Design review of the part built by this model. Coordinates are the model's own, in mm. Face numbers are marked on the shaded views. A direction names the side the tool comes from. Coordinates: 2 decimals unless noted, no trailing zeros. Loops run counter-clockwise (first coordinate to the right, second up) from the corner with the lowest first, then second, coordinate; pieces in that order, holes last. Notation, with made-up numbers: M -21.5,-23.75 L 34.5,-23.75 A21 cw 34.5,15.25 Z; hole C 23.5,5 d6. An arc over 180 degrees is marked long. One line per item, written item: value.
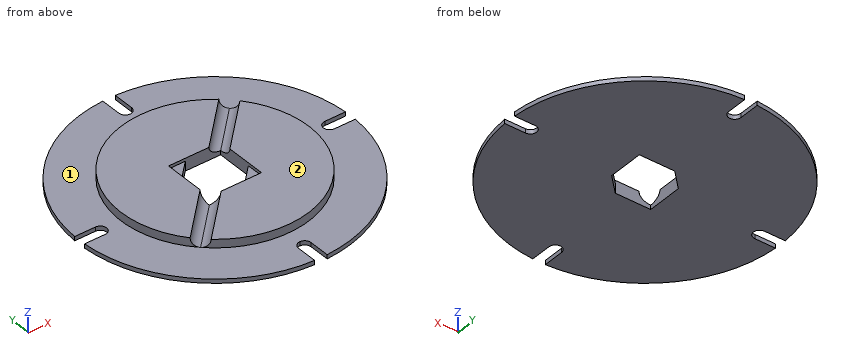
```python
from build123d import *

# Parameters (mm, degrees)
F2_DEPTH      = 2
F3_DEPTH      = 6
F4_DEPTH      = 6
F5_DEPTH      = 4.6
F9_DEPTH      = 45
F9_DEPTH_BACK = 45


with BuildPart() as f2:
    # F0 (on Top) → F2 (new body)
    with BuildSketch(Plane.XY):
        with BuildLine():
            Line((55, 3), (64.930732323, 3))
            ThreePointArc((64.930732323, 3), (45.9619407771, 45.9619407771), (3, 64.930732323))
            Line((3, 64.930732323), (3, 55))
            ThreePointArc((3, 55), (0, 52), (-3, 55))
            Line((-3, 55), (-3, 64.930732323))
            ThreePointArc((-3, 64.930732323), (-45.9619407771, 45.9619407771), (-64.930732323, 3))
            Line((-64.930732323, 3), (-55, 3))
            ThreePointArc((-55, 3), (-52, 0), (-55, -3))
            Line((-55, -3), (-64.930732323, -3))
            ThreePointArc((-64.930732323, -3), (-45.9619407771, -45.9619407771), (-3, -64.930732323))
            Line((-3, -64.930732323), (-3, -55))
            ThreePointArc((-3, -55), (-2.1213203436, -52.8786796564), (0, -52))
            ThreePointArc((0, -52), (2.1213203436, -52.8786796564), (3, -55))
            Line((3, -55), (3, -64.930732323))
            ThreePointArc((3, -64.930732323), (45.9619407771, -45.9619407771), (64.930732323, -3))
            Line((64.930732323, -3), (55, -3))
            ThreePointArc((55, -3), (52, 0), (55, 3))
        make_face()
        with BuildLine():
            ThreePointArc((45, 0), (31.8198051534, -31.8198051534), (0, -45))
            ThreePointArc((0, -45), (-31.8198051534, 31.8198051534), (45, 0))
        make_face(mode=Mode.SUBTRACT)
    extrude(amount=F2_DEPTH)

    # F0 (on Top) → F3 (join)
    with BuildSketch(Plane.XY):
        with BuildLine():
            ThreePointArc((45, 0), (-31.8198051534, 31.8198051534), (0, -45))
            ThreePointArc((0, -45), (31.8198051534, -31.8198051534), (45, 0))
        make_face()
    extrude(amount=F3_DEPTH)

    # F1 (on Top) → F4 (cut)
    with BuildSketch(Plane.XY):
        Polygon((4.4705627485, -12.5), (12.5, -12.5), (12.5, -4.4705627485), align=None)
        with BuildLine():
            Line((-12.5, -12.5), (4.4705627485, -12.5))
            Line((4.4705627485, -12.5), (12.5, -4.4705627485))
            Line((12.5, -4.4705627485), (12.5, 12.5))
            Line((12.5, 12.5), (7.4246212025, 7.4246212025))
            ThreePointArc((7.4246212025, 7.4246212025), (9.7007350914, 4.0181760398), (10.5, 0))
            ThreePointArc((10.5, 0), (4.0181760398, -9.7007350914), (-7.4246212025, -7.4246212025))
            Line((-7.4246212025, -7.4246212025), (-12.5, -12.5))
        make_face()
        with BuildLine():
            Line((-12.5, 4.4705627485), (-12.5, -12.5))
            Line((-12.5, -12.5), (-7.4246212025, -7.4246212025))
            ThreePointArc((-7.4246212025, -7.4246212025), (-7.4246212025, 7.4246212025), (7.4246212025, 7.4246212025))
            Line((7.4246212025, 7.4246212025), (12.5, 12.5))
            Line((12.5, 12.5), (-4.4705627485, 12.5))
            Line((-4.4705627485, 12.5), (-12.5, 4.4705627485))
        make_face()
        Polygon((-12.5, 12.5), (-12.5, 4.4705627485), (-4.4705627485, 12.5), align=None)
        with BuildLine():
            Line((7.4246212025, 7.4246212025), (-7.4246212025, -7.4246212025))
            ThreePointArc((-7.4246212025, -7.4246212025), (4.0181760398, -9.7007350914), (10.5, 0))
            ThreePointArc((10.5, 0), (9.7007350914, 4.0181760398), (7.4246212025, 7.4246212025))
        make_face()
        with BuildLine():
            ThreePointArc((7.4246212025, 7.4246212025), (-7.4246212025, 7.4246212025), (-7.4246212025, -7.4246212025))
            Line((-7.4246212025, -7.4246212025), (7.4246212025, 7.4246212025))
        make_face()
    extrude(amount=F4_DEPTH, mode=Mode.SUBTRACT)

    # F1 (on Top) → F5 (join)
    with BuildSketch(Plane.XY):
        Polygon((-12.5, 12.5), (-12.5, 4.4705627485), (-4.4705627485, 12.5), align=None)
        Polygon((4.4705627485, -12.5), (12.5, -12.5), (12.5, -4.4705627485), align=None)
    extrude(amount=F5_DEPTH)

    # F8 (on line) → F9 (cut, two sides)
    with BuildSketch(Plane(origin=(0, 0, 0), x_dir=(-0.7071067812, 0.7071067812, 0), z_dir=(0.7071067812, 0.7071067812, 0))) as f9_sk:
        with BuildLine():
            ThreePointArc((0, 2), (2.8284271247, 3.1715728753), (4, 6))
            ThreePointArc((4, 6), (-2.8284271247, 8.8284271247), (0, 2))
        make_face()
    extrude(amount=-F9_DEPTH, mode=Mode.SUBTRACT)
    extrude(f9_sk.sketch, amount=F9_DEPTH_BACK, mode=Mode.SUBTRACT)


solid = f2.part
```
(1) We need section B-B on z = 3.25. State the section outline as (x, y) points, then the cut area to 3 significant figures.
Reply:
outline: M -33.81,-29.7 L -12.5,-8.39 L -12.5,4.47 L -4.47,12.5 L 8.39,12.5 L 29.7,33.81 A45 ccw Z; M -29.7,-33.81 A45 ccw 33.81,29.7 L 12.5,8.39 L 12.5,-4.47 L 4.47,-12.5 L -8.39,-12.5 Z
area: 5,470 mm2
(2) Insertion check: pin 1 (1.6 mm diameter, centred on y = 58.5, z = 1.5, fed in from +X); pin 2 (1.8 mm diameter, centred on y = -4, z = 3.5, fed in from +X); pin 3 (3 mm diameter, centred on y = 5.5, z = 4, fed in from -X). Each pin has a flat end and moves straight along its axis. Give the tip position at first contact, or say it passes through.
Reply:
pin 1: stops at x = 29.93
pin 2: stops at x = 44.89
pin 3: stops at x = -44.82
(3) We need section A-A on y = -53.5. State the section outline as (x, z) points.
Reply:
outline: M -36.92,0 L -2.6,0 L -2.6,2 L -36.92,2 Z; M 2.6,0 L 36.92,0 L 36.92,2 L 2.6,2 Z
(4) To check wall thickness, follow line 1 along Y through (x, z) = (7.5, 1); line 2 along Y through (x, z) = (-24.5, 5); line 3 along X through (y, z) = (29, 4). State the ranges of each line that lie inside material, in increasing order. Write a range as [from, to].
Reply:
line 1: y = [-64.57, -9.47], [12.5, 64.57]
line 2: y = [-37.75, -29.98], [-19.02, 37.75]
line 3: x = [-34.41, 24.1], [33.9, 34.41]
(5) Tool access review of the marked faces 1 and 2: name each direction out of +Z, -Z, +X, -X, +Y, -Y from which nothing blocks a thin tool from reaching the whole face with its end or side.
Reply:
face 1: +Z
face 2: +Z, +X, -X, +Y, -Y
(6) We need section C-C on x = -48.5. State the section outline as (y, z) points, then the cut area to 3 significant figures.
Reply:
outline: M -43.28,0 L 43.28,0 L 43.28,2 L -43.28,2 Z
area: 173 mm2
